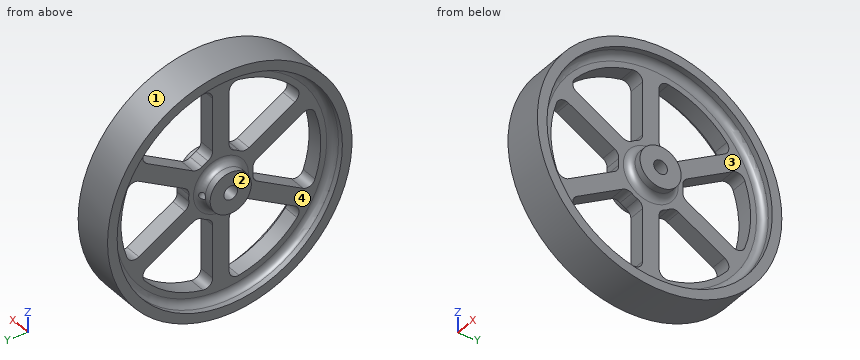
Autodesk Inventor part; units mm, degrees
ref_plane "Arbeitsebene1" through (0, 0, 0) normal (0.5, -0.866, 0) x (0, 0, 1)
ref_plane "XZ Plane" through (0, 0, 0) normal (0, 1, 0) x (-1, 0, 0)
ref_plane "XY Plane" through (0, 0, 0) normal (0, 0, 1) x (1, 0, 0)
sketch "Skizze2" plane through (0, 0, 0) normal (0, 0, 1) x (1, 0, 0)
  line L0 (0, -21.0687) -> (0, 71.4095)
  line L1 (-11.2, 0) -> (11.2, 0)
  line L2 (-8, 2.5) -> (-8, 7.5)
  line L3 (-5.5, 7.5) -> (-8, 7.5)
  arc A0 (-5.5, 7.5) -> (-3, 10) centre (-5.5, 10) ccw
  line L4 (-3, 10) -> (-3, 38.5)
  arc A1 (-3, 38.5) -> (-5.5, 41) centre (-5.5, 38.5) ccw
  line L5 (-7.5, 44.5) -> (7.5, 44.5)
  line L6 (7.5, 44.5) -> (7.5, 41)
  line L7 (7.5, 41) -> (5.5, 41)
  arc A2 (5.5, 41) -> (3, 38.5) centre (5.5, 38.5) ccw
  line L8 (3, 38.5) -> (3, 10)
  arc A3 (3, 10) -> (5.5, 7.5) centre (5.5, 10) ccw
  line L9 (5.5, 7.5) -> (8, 7.5)
  line L10 (8, 7.5) -> (8, 2.5)
  line L11 (-8, 2.5) -> (8, 2.5)
  line L12 (-7.5, 44.5) -> (-7.5, 41)
  line L13 (-7.5, 41) -> (-5.5, 41)
  line L14 (0, 58.1983) -> (0, -7.8576) construction
  point P0 (0, 0)
  dimension "d5" = 15
  dimension "d7" = 2.5
  dimension "d8" = 2.5
  dimension "d9" = 2.5
  dimension "d10" = 2.5
  dimension "d11" = 89
  dimension "d12" = 82
  dimension "d13" = 15
  dimension "d14" = 6
  dimension "d15" = 7.5
  dimension "d16" = 5
  dimension "d41" = 16
revolve "Umdrehung1" add sketch "Skizze2" angle 360 about axis through (-10, 0, 0) along (1, 0, 0)
sketch "Skizze3" plane through (-3, 0, 0) normal (-1, 0, 0) x (0, 0, 1)
  line L0 (0, -62.3) -> (0, 62.3)
  line L1 (-62.3, 0) -> (62.3, 0)
  line L2 (-3.0822, 11.3385) -> (-15.5149, 32.8726)
  line L3 (3.0822, 11.3385) -> (15.5149, 32.8726)
  line L4 (-8.2784, 8.3385) -> (-20.7111, 29.8726)
  line L5 (-36.226, 3) -> (-11.3606, 3)
  line L6 (11.3606, 3) -> (36.226, 3)
  line L7 (8.2784, 8.3385) -> (20.7111, 29.8726)
  line L8 (-3.0822, -11.3385) -> (-15.5149, -32.8726)
  line L9 (3.0822, -11.3385) -> (15.5149, -32.8726)
  line L10 (-8.2784, -8.3385) -> (-20.7111, -29.8726)
  line L11 (-36.226, -3) -> (-11.3606, -3)
  line L12 (11.3606, -3) -> (36.226, -3)
  line L13 (8.2784, -8.3385) -> (20.7111, -29.8726)
  arc A0 (3.0822, 11.3385) -> (-3.0822, 11.3385) centre (0, 0) ccw
  arc A1 (15.5149, 32.8726) -> (-15.5149, 32.8726) centre (0, 0) ccw
  arc A2 (36.226, 3) -> (20.7111, 29.8726) centre (0, 0) ccw
  arc A3 (-20.7111, 29.8726) -> (-36.226, 3) centre (0, 0) ccw
  arc A4 (20.7111, -29.8726) -> (36.226, -3) centre (0, 0) ccw
  arc A5 (-36.226, -3) -> (-20.7111, -29.8726) centre (0, 0) ccw
  arc A6 (-15.5149, -32.8726) -> (15.5149, -32.8726) centre (0, 0) ccw
  arc A7 (-8.2784, 8.3385) -> (-11.3606, 3) centre (0, 0) ccw
  arc A8 (-11.3606, -3) -> (-8.2784, -8.3385) centre (0, 0) ccw
  arc A9 (-3.0822, -11.3385) -> (3.0822, -11.3385) centre (0, 0) ccw
  arc A10 (8.2784, -8.3385) -> (11.3606, -3) centre (0, 0) ccw
  arc A11 (11.3606, 3) -> (8.2784, 8.3385) centre (0, 0) ccw
  dimension "d21" = 60
  dimension "d23" = 6
  dimension "d24" = 6
  dimension "d25" = 3
  dimension "d26" = 3
  dimension "d27" = 60
  dimension "d28" = 36.35
  dimension "d29" = 11.75
  dimension "d30" = 36.35
  dimension "d31" = 11.75
  dimension "d32" = 36.35
  dimension "d33" = 11.75
extrude "Extrusion2" cut sketch "Skizze3" against normal through all
fillet "Rundung1" radius 3 4 edges at (0, 11.3385, -3.0822) (0, 11.3385, 3.0822) (0, 32.8726, -15.5149) (0, 32.8726, 15.5149)
pattern_circular "Runde Anordnung1" count 6 over 360 about axis through (-6.75, 0, 0) along (1, 0, 0) of "Rundung1"
ref_plane "Arbeitsebene1" through (0, 0, 0) normal (0.5, -0.866, 0) x (0, 0, 1)
sketch "Skizze5" plane through (0, 0, 0) normal (0.5, -0.866, 0) x (0, 0, 1)
  point P0 (0, 0)
  point P1 (0, 0)
hole "Bohrung1" at (0, 0, 0) direction (-0.5, 0.866, 0) diameter 2.459 depth 10 tip angle 118
properties part number "Schwungrad"
Geometry: final body of the model. Coordinates: model frame, mm. Face numbers are marked on the shaded views. Round coordinates to 2 decimals unless told otherwise and drop trailing zeros.
Item 1: Section query B-B (y = -24). Give the number of separate pieces and of enclosed holes in the cut face, plus the area to 3 significant figures.
Item 2: Material intervals for L1, parallel to Z at x = -6.45, y = 0; L2, parallel to Z at x = 3.5, y = -4; L3, parallel to Y at x = -0.25, z = 6, sorted ascending.
Item 3: Mould query, pull axis Z, two halves, no side actions, for the marked faces 1, 2, 3 and 4. Classes: +Z half, -Z half, draft (parallel to the pull), parting line (faces both ways), or undercut.
Item 4: Pin query (flat end, axial travel): P1, Ø6.5, axis at x = -1, z = -27, coming from the -Y side; P2, Ø1, axis at x = -2.5, y = 12, coming from the +Z side; P3, Ø4, axis at x = 1, z = 13.5, coming from the +Y side; P4, Ø8, axis at x = -3, z = 2, coming from the +Y side. Return the tip coordinate at first contact, or that it passes through.
Completed:
1. separate pieces: 4
1. enclosed holes: 0
1. area: 288 mm2
2. L1: z = -44.5 to -41, -7.5 to -2.5, 2.5 to 7.5, 41 to 44.5
2. L2: z = -44.32 to -39.8, -7.5 to 7.5, 39.8 to 44.32
2. L3: y = -44.09 to -35.85, -16.39 to 16.39, 35.85 to 44.09
3. face 1: parting line
3. face 2: draft
3. face 3: undercut
3. face 4: undercut
4. P1: stops at y = -37.63
4. P2: stops at z = 42.99
4. P3: stops at y = 42.99
4. P4: stops at y = 44.5
